The listing builds one solid part. Answer for the finished solid, in the listing's coordinates (mm). Face numbers are marked on the shaded views. A direction names the side the tool comes from. Round coordinates to 2 decimals unless told otherwise and drop trailing zeros. Loops run counter-clockwise (first coordinate to the right, second up) from the corner with the lowest first, then second, coordinate; pieces in that order, holes last. Notation, with made-up numbers: M -16.75,-26.5 L -5.75,-26.5 A24 ccw -5.75,-12.5 Z; hole C 71.25,62 d8. An arc over 180 degrees is marked long. Put each result on its own line as item: value. Start each with the question number.
(1) Determine the mould class of the marked faces 1, 2, 3 and 4 for opening direction X: released by +X, released by -X, zero draft, split by the parting line, or undercut.
(2) Section C-C, the plane y = -31 is taken. Determine the outline of the cut face in (x, z), then the cut area to 3 significant figures.
(3) Section B-B, the plane z = 35 is taken. Determine the outline of the cut face in (x, y), then the cut area to 3 significant figures.
(4) Flat-ended cylindrical pins translate along their axes: P1, Ø3, axis at x = 34, y = -19, coming from the -Z side; P2, Ø10, axis at x = 35.5, z = 62, coming from the -Y side; P3, Ø6, axis at y = -37, z = 46.5, coming from the -X side. Find the tip coordinate at first contact, or state that the pin passes through.
(5) Which of the six approach directions +Z, -Z, +X, -X, +Y, -Y give full straight-line access (tool end or side, diameter ignored) to the marked faces 5 and 6?
(6) Section A-A, the plane x = 25 is taken. Determine the outline of the cut face in (y, z).
(7) Section D-D, the plane x = 79.5 is taken. Determine the outline of the cut face in (y, z).
(8) Straight lines are drawn through the part: line 1 (X direction, y = -39, z = 30); line 2 (Y direction, x = 18, z = 49); line 3 (X direction, y = -26, z = 37). For each, find the intervals that lie inside material, in ascending order.
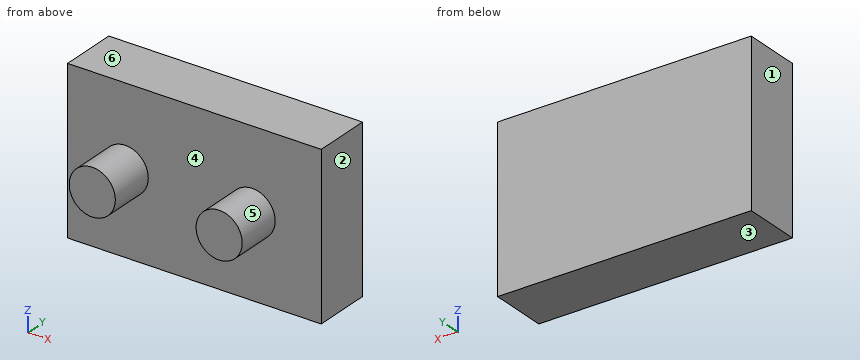
```python
from build123d import *

# Parameters (mm, degrees)
F0_W     = 110
F0_H     = 70
F1_DEPTH = 25
F2_R     = 10
F3_DEPTH = 20


with BuildPart() as f1:
    # F0 (on Front) → F1 (new body)
    with BuildSketch(Plane.XZ):
        with Locations((55, 35)):
            Rectangle(F0_W, F0_H)
    extrude(amount=F1_DEPTH)

    # F2 (on face) → F3 (join)
    with BuildSketch(Plane.XZ.offset(25)):
        with Locations((25, 35)):
            Circle(F2_R)
        with BuildLine():
            ThreePointArc((90, 35), (80, 45), (70, 35))
            ThreePointArc((70, 35), (80, 25), (90, 35))
        make_face()
    extrude(amount=F3_DEPTH)


solid = f1.part
```
Recorded:
1. face 1: released by -X
1. face 2: released by +X
1. face 3: zero draft
1. face 4: undercut
2. outline: C 25,35 d20; C 80,35 d20
2. area: 628 mm²
3. outline: M 0,-25 L 15,-25 L 15,-45 L 35,-45 L 35,-25 L 70,-25 L 70,-45 L 90,-45 L 90,-25 L 110,-25 L 110,0 L 0,0 Z
3. area: 3,550 mm²
4. P1: stops at z = 0
4. P2: stops at y = -25
4. P3: stops at x = 19.73
5. face 5: -Y
5. face 6: +Z, +X, -X, +Y, -Y
6. outline: M -45,25 L -25,25 L -25,0 L 0,0 L 0,70 L -25,70 L -25,45 L -45,45 Z
7. outline: M -45,25.01 L -25,25.01 L -25,0 L 0,0 L 0,70 L -25,70 L -25,44.99 L -45,44.99 Z
8. line 1: x = 16.34 to 33.66, 71.34 to 88.66
8. line 2: y = -25 to 0
8. line 3: x = 15.2 to 34.8, 70.2 to 89.8
